The listing builds one solid part. Answer for the finished solid, in the listing's coordinates (mm). A direction names the side the tool comes from. Round coordinates to 2 decimals unless told otherwise and drop trailing zeros. Write each loop counter-clockwise with the first axis right and the second up, starting at its lowest first coordinate (ties: lowest second). Pieces come first, ordered by that corner, then holes. Notation, with made-up numbers: (12.5, 9) - (66.5, 9) arc R24 cw to (66.5, 46) - close; hole circle Ø5 at (-4, -24.75). An arc over 180 degrees is marked (long way). Return JSON: item names as keys, results as strings. Group by question number.
from build123d import *

# Parameters (mm, degrees)
BOSS_EXTRUDE1_DEPTH   = 550
F_4_0MM_DOWEL_HOLE1_D = 4
CUT_EXTRUDE1_DEPTH    = 582.946448297


with BuildPart() as part:
    # Sketch1 → Boss-Extrude1 (new body)
    with BuildSketch(Plane.XY):
        Polygon((-175.647058824, 7.852941176), (-175.647058824, -7.147058824), (14.352941176, -7.147058824), (14.352941176, 7.852941176), (9.352941176, 7.852941176), (9.352941176, -6.147058824), (-170.647058824, -6.147058824), (-170.647058824, 7.852941176), align=None)
    extrude(amount=BOSS_EXTRUDE1_DEPTH)

    # Ø4.0mm Dowel Hole1 (through all)
    with Locations(Plane(origin=(14.352941176, 0, 0), x_dir=(0, 0, -1), z_dir=(1, 0, 0))):
        with Locations((-540, -0.147058824)):
            Hole(F_4_0MM_DOWEL_HOLE1_D / 2)

    # Sketch5 → Cut-Extrude1 (cut, through all)
    with BuildSketch(Plane(origin=(14.352941176, 0, 0), x_dir=(0, 0, -1), z_dir=(1, 0, 0))):
        with BuildLine():
            Line((-65, 1.852941176), (-15, 1.852941176))
            ThreePointArc((-15, 1.852941176), (-13, -0.147058824), (-15, -2.147058824))
            Line((-15, -2.147058824), (-65, -2.147058824))
            ThreePointArc((-65, -2.147058824), (-67, -0.147058824), (-65, 1.852941176))
        make_face()
    extrude(amount=-CUT_EXTRUDE1_DEPTH, mode=Mode.SUBTRACT)


solid = part.part
(1) For faces 1 (the flat face through (14.353, 0, 271)), 2 (the flat face through (9.353, 1, 271)), determine the directions among +Z, -Z, +X, -X, +Y, -Y from which every point of the face is accessible in a straight line to the end or side of a thin tool.
(2) Find section A-A (y = 4.25). Write down the section's boundary in (x, z).
(3) Find section D-D (x = -27.5). Write down the section's boundary in (y, z), plus the area to 3 significant figures.
(4) Find section B-B (z = 43). Write down the section's boundary in (x, y).
(5) Find section C-C (z = 181). Write down the section's boundary in (x, y).
(6) Consider line 1 (X direction, y = 6.25, z = 267); line 2 (Y direction, x = -172.45, z = 540); line 3 (Y direction, x = -116, z = 290). Determine where each line is inside the solid, lowest interval first.
Check sheet entries:
{
 "1": {"face 1": "+Z, -Z, +X, +Y, -Y", "face 2": "+Z, -Z, +Y"},
 "2": {"outline": "(-175.65, 0) - (-170.65, 0) - (-170.65, 550) - (-175.65, 550) - close; (9.35, 0) - (14.35, 0) - (14.35, 550) - (9.35, 550) - close"},
 "3": {"outline": "(-7.15, 0) - (-6.15, 0) - (-6.15, 550) - (-7.15, 550) - close", "area": "550 mm^2"},
 "4": {"outline": "(-175.65, -7.15) - (14.35, -7.15) - (14.35, -2.15) - (9.35, -2.15) - (9.35, -6.15) - (-170.65, -6.15) - (-170.65, -2.15) - (-175.65, -2.15) - close; (-175.65, 1.85) - (-170.65, 1.85) - (-170.65, 7.85) - (-175.65, 7.85) - close; (9.35, 1.85) - (14.35, 1.85) - (14.35, 7.85) - (9.35, 7.85) - close"},
 "5": {"outline": "(-175.65, -7.15) - (14.35, -7.15) - (14.35, 7.85) - (9.35, 7.85) - (9.35, -6.15) - (-170.65, -6.15) - (-170.65, 7.85) - (-175.65, 7.85) - close"},
 "6": {"line 1": "x = -175.65 to -170.65, 9.35 to 14.35", "line 2": "y = -7.15 to -2.15, 1.85 to 7.85", "line 3": "y = -7.15 to -6.15"}
}
